from build123d import *

# Parameters (mm, degrees)
F1_DEPTH = 57.15
F3_R     = 6.35
F2_R     = 6.35
F4_DEPTH = 12.7


with BuildPart() as f1:
    # F0 (on Front) → F1 (new body)
    with BuildSketch(Plane.XZ):
        with BuildLine():
            Line((-76.2, -22.225), (76.2, -22.225))
            Line((76.2, -22.225), (76.2, -9.525))
            Line((76.2, -9.525), (44.45, -9.525))
            Line((44.45, -9.525), (44.45, 22.225))
            Line((44.45, 22.225), (31.75, 22.225))
            ThreePointArc((31.75, 22.225), (0, -9.525), (-31.75, 22.225))
            Line((-31.75, 22.225), (-44.45, 22.225))
            Line((-44.45, 22.225), (-44.45, -9.525))
            Line((-44.45, -9.525), (-76.2, -9.525))
            Line((-76.2, -9.525), (-76.2, -22.225))
        make_face()
    extrude(amount=F1_DEPTH)

    # F3 (on face) + F2 (on face) → F4 (cut)
    with BuildSketch(Plane.XY.offset(-9.525)):
        with Locations((-60.325, -28.575)):
            Circle(F3_R)
    with BuildSketch(Plane.XY.offset(-9.525)):
        with Locations((60.325, -28.575)):
            Circle(F2_R)
    extrude(amount=-F4_DEPTH, mode=Mode.SUBTRACT)


solid = f1.part
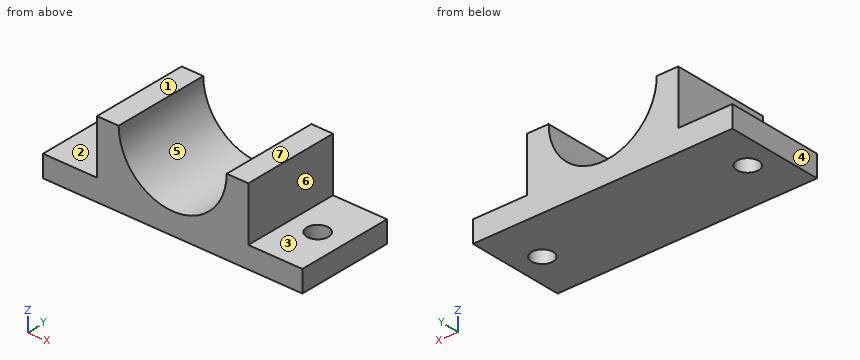
Build history of the part. All positions in model axes, mm. Face numbers are marked on the shaded views. A direction names the side the tool comes from. Round coordinates to 2 decimals unless told otherwise and drop trailing zeros. Loops run counter-clockwise (first coordinate to the right, second up) from the corner with the lowest first, then second, coordinate; pieces in that order, holes last. Notation, with made-up numbers: (-39, -3.5) -> (-34, -3.5) arc R31 cw to (-34, 33.5) -> close; hole circle Ø6 at (12.5, 12.5). An arc over 180 degrees is marked (long way). Answer in a Markdown table with one row per item.
Item 1: Saw through at C-C (y = -48). Write the cut outline in (x, z) (3 decimals).
Answers below:
| item | result |
|---|---|
| outline | (-76.2, -22.225) -> (76.2, -22.225) -> (76.2, -9.525) -> (44.45, -9.525) -> (44.45, 22.225) -> (31.75, 22.225) arc R31.75 cw to (-31.75, 22.225) -> (-44.45, 22.225) -> (-44.45, -9.525) -> (-76.2, -9.525) -> close |
Item 2: Which spindle directions (+Z, -Z, +X, -X, +Y, -Y) get a long thin tool onto all of the face, cutting with end or side? Do the marked faces 1, 2 and 3. Say none if no direction does.
Answers below:
| item | result |
|---|---|
| face 1 | +Z, +X, -X, +Y, -Y |
| face 2 | +Z, -X, +Y, -Y |
| face 3 | +Z, +X, +Y, -Y |
Item 3: Saw through at B-B (z = 7). Write the cut outline in (x, y).
Answers below:
| item | result |
|---|---|
| outline | (-44.45, -57.15) -> (-27.86, -57.15) -> (-27.86, 0) -> (-44.45, 0) -> close; (27.86, -57.15) -> (44.45, -57.15) -> (44.45, 0) -> (27.86, 0) -> close |
Item 4: Mould opens along X. For the marked faces 4, 5, 6 and 7 say: +X half, -X half, draft (parallel to the pull), parting line (faces both ways), or undercut.
Answers below:
| item | result |
|---|---|
| face 4 | -X half |
| face 5 | undercut |
| face 6 | +X half |
| face 7 | draft |
Item 5: Drill centre lines: L1, parallel to Z at x = -51.5, y = -30 (3 decimals); L2, parallel to X at y = -8, z = 7; L3, parallel to X at y = -54, z = -3.5. Where is each one in solid material? Low to high. Write a range as [from, to].
Answers below:
| item | result |
|---|---|
| L1 | z = [-22.225, -9.525] |
| L2 | x = [-44.45, -27.86], [27.86, 44.45] |
| L3 | x = [-44.45, -18.61], [18.61, 44.45] |
Item 6: Saw through at D-D (x = -16.5). Write the cut outline in (y, z) (3 decimals), and give its area (3 significant figures).
Answers below:
| item | result |
|---|---|
| outline | (-57.15, -22.225) -> (0, -22.225) -> (0, -4.901) -> (-57.15, -4.901) -> close |
| area | 990 mm² |
Item 7: Pin check, flat tips, straight feed: pin 1 (9.5 mm diameter, centred on x = 65, y = -14.5, fed in from +Z) (3 decimals); pin 2 (3 mm diameter, centred on y = -22, z = 14, fed in from -X); pin 3 (11.5 mm diameter, centred on x = -60.325, y = -28.575, fed in from +Z); pin 4 (6 mm diameter, centred on y = -6, z = 7, fed in from +X). Stop position of each tip, or through.
Answers below:
| item | result |
|---|---|
| pin 1 | stops at z = -9.525 |
| pin 2 | stops at x = -44.45 |
| pin 3 | passes through |
| pin 4 | stops at x = 44.45 |
Item 8: Saw through at A-A (y = -32.5). Write the cut outline in (x, z) (3 decimals).
Answers below:
| item | result |
|---|---|
| outline | (-76.2, -22.225) -> (-65.317, -22.225) -> (-65.317, -9.525) -> (-76.2, -9.525) -> close; (-55.333, -22.225) -> (55.333, -22.225) -> (55.333, -9.525) -> (44.45, -9.525) -> (44.45, 22.225) -> (31.75, 22.225) arc R31.75 cw to (-31.75, 22.225) -> (-44.45, 22.225) -> (-44.45, -9.525) -> (-55.333, -9.525) -> close; (65.317, -22.225) -> (76.2, -22.225) -> (76.2, -9.525) -> (65.317, -9.525) -> close |
